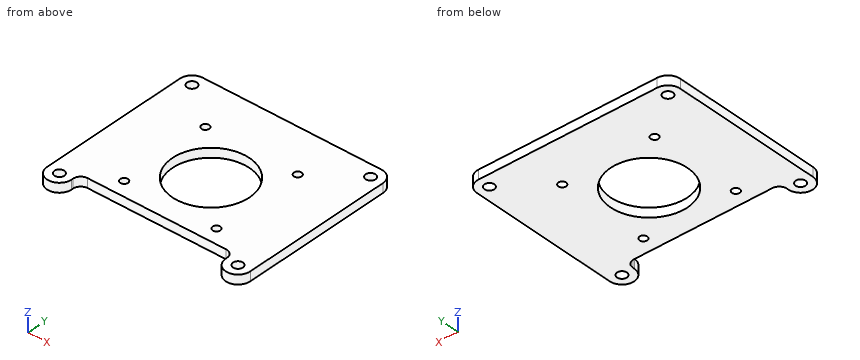
from build123d import *

# Parameters (mm, degrees)
SKETCH_1_R          = 1.6
EXTRUDE_1_DEPTH     = 3
SKETCH_2_R          = 1.25
SKETCH_2_R_2        = 12.5
CUT_EXTRUDE_1_DEPTH = 60.983331018


with BuildPart() as part:
    # ｽｹｯﾁ1 → ﾎﾞｽ - 押し出し1 (new body)
    with BuildSketch(Plane.XY):
        with BuildLine():
            Line((22.5, 0), (-22.5, 0))
            ThreePointArc((-22.5, 0), (-24.267766953, -0.732233047), (-25, -2.5))
            Line((-25, -2.5), (-25, -3))
            ThreePointArc((-25, -3), (-29, -7), (-33, -3))
            Line((-33, -3), (-33, 46))
            ThreePointArc((-33, 46), (-31.828427125, 48.828427125), (-29, 50))
            Line((-29, 50), (29, 50))
            ThreePointArc((29, 50), (31.828427125, 48.828427125), (33, 46))
            Line((33, 46), (33, -3))
            ThreePointArc((33, -3), (29, -7), (25, -3))
            Line((25, -3), (25, -2.5))
            ThreePointArc((25, -2.5), (24.267766953, -0.732233047), (22.5, 0))
        make_face()
        with Locations((-29, -3)):
            Circle(SKETCH_1_R, mode=Mode.SUBTRACT)
        with Locations((-29, 46)):
            Circle(SKETCH_1_R, mode=Mode.SUBTRACT)
        with Locations(Location((29, 46, 0), (0, 0, 180))):
            Circle(SKETCH_1_R, mode=Mode.SUBTRACT)
        with Locations(Location((29, -3, 0), (0, 0, 180))):
            Circle(SKETCH_1_R, mode=Mode.SUBTRACT)
    extrude(amount=EXTRUDE_1_DEPTH)

    # ｽｹｯﾁ2 → ｶｯﾄ - 押し出し1 (cut, through all)
    with BuildSketch(Plane.XY.offset(3)):
        with Locations((-15, 35)):
            Circle(SKETCH_2_R)
        with Locations((-15, 5)):
            Circle(SKETCH_2_R)
        with Locations((15, 5)):
            Circle(SKETCH_2_R)
        with Locations((15, 35)):
            Circle(SKETCH_2_R)
        with Locations((0, 20)):
            Circle(SKETCH_2_R_2)
    extrude(amount=-CUT_EXTRUDE_1_DEPTH, mode=Mode.SUBTRACT)


solid = part.part
Geometry: final body of the model. Coordinates: model frame, mm. Coordinates: 2 decimals unless noted, no trailing zeros. Order: outer loops, then holes, each group sorted by start corner. A loop starts at its lowest first (then second) coordinate and runs counter-clockwise, first axis right, second up.
(1) Section query A-A (x = -15). Return the cut outline in (y, z).
(2) First-contact query: pin 1 (1.9 mm diameter, centred on x = -29, y = -3, fed in from -Z). Flat tip, straight axial feed; report the tip coordinate or a pass-through.
(3) Material intervals for probe 1 along Y at (x, z) = (-29, 0.65); probe 2 along Y at (x, z) = (-15, 2.35); probe 3 along X at (y, z) = (6, 1.2), sorted ascending.
(4) Section query C-C (z = 1.1). State how many separate pieces and enclosed holes the cut face has, plus the area to 3 significant figures.
(5) Section query B-B (y = 20). Return the cut outline in (x, z), plus the area to 3 significant figures.
(6) Section query D-D (y = 5). Return the cut outline in (x, z).
Solution:
1. outline: (0, 0) - (3.75, 0) - (3.75, 3) - (0, 3) - close; (6.25, 0) - (33.75, 0) - (33.75, 3) - (6.25, 3) - close; (36.25, 0) - (50, 0) - (50, 3) - (36.25, 3) - close
2. pin 1: passes through
3. probe 1: y = -7 to -4.6, -1.4 to 44.4, 47.6 to 50
3. probe 2: y = 0 to 3.75, 6.25 to 33.75, 36.25 to 50
3. probe 3: x = -33 to -15.75, -14.25 to 14.25, 15.75 to 33
4. separate pieces: 1
4. enclosed holes: 9
4. area: 2,850 mm2
5. outline: (-33, 0) - (-12.5, 0) - (-12.5, 3) - (-33, 3) - close; (12.5, 0) - (33, 0) - (33, 3) - (12.5, 3) - close
5. area: 123 mm2
6. outline: (-33, 0) - (-16.25, 0) - (-16.25, 3) - (-33, 3) - close; (-13.75, 0) - (13.75, 0) - (13.75, 3) - (-13.75, 3) - close; (16.25, 0) - (33, 0) - (33, 3) - (16.25, 3) - close
